from build123d import *

# Parameters (mm, degrees)
IZIM1_W                     = 30
IZIM1_H                     = 30
Y_KSEKLIK_EKSTR_ZYON1_DEPTH = 8
IZIM3_R                     = 1.75
KES_EKSTR_ZYON1_DEPTH       = 30
Y_KSEKLIK_EKSTR_ZYON3_DEPTH = 30
KES_EKSTR_ZYON2_DEPTH       = 30
IZIM5_R                     = 4.15
KES_EKSTR_ZYON3_DEPTH       = 30
IZIM6_W                     = 3
IZIM6_H                     = 1.5


with BuildPart() as part:
    # Çizim1 → Yükseklik-Ekstrüzyon1 (new body)
    with BuildSketch(Plane.XY):
        with Locations((15, 15)):
            Rectangle(IZIM1_W, IZIM1_H)
    extrude(amount=Y_KSEKLIK_EKSTR_ZYON1_DEPTH)

    # Çizim3 → Kes-Ekstrüzyon1 (cut)
    with BuildSketch(Plane.XY.offset(8)):
        with Locations((4, 26)):
            Circle(IZIM3_R)
        with Locations((4, 4)):
            Circle(IZIM3_R)
        with Locations((26, 26)):
            Circle(IZIM3_R)
        with Locations((26, 4)):
            Circle(IZIM3_R)
    extrude(amount=-KES_EKSTR_ZYON1_DEPTH, mode=Mode.SUBTRACT)

    # Çizim2 → Yükseklik-Ekstrüzyon3 (add)
    with BuildSketch(Plane.XY.offset(8)):
        with BuildLine():
            Line((6.161165235, 6.161165235), (9.590633124, 9.590633124))
            ThreePointArc((9.590633124, 9.590633124), (9.590633124, 20.409366876), (20.409366876, 20.409366876))
            Line((20.409366876, 20.409366876), (23.838834765, 23.838834765))
            ThreePointArc((23.838834765, 23.838834765), (6.161165235, 23.838834765), (6.161165235, 6.161165235))
        make_face()
    extrude(amount=Y_KSEKLIK_EKSTR_ZYON3_DEPTH)

    # Çizim4 → Kes-Ekstrüzyon2 (cut)
    with BuildSketch(Plane.XY.offset(8)):
        with BuildLine():
            Line((0, 15), (0, 30))
            Line((0, 30), (15, 30))
            ThreePointArc((15, 30), (6.161165235, 23.838834765), (0, 15))
        make_face()
    extrude(amount=-KES_EKSTR_ZYON2_DEPTH, mode=Mode.SUBTRACT)

    # Çizim5 → Kes-Ekstrüzyon3 (cut)
    with BuildSketch(Plane.XY.offset(8)):
        with Locations((15, 15)):
            Circle(IZIM5_R)
    extrude(amount=-KES_EKSTR_ZYON3_DEPTH, mode=Mode.SUBTRACT)

    # Çizim6 → Kes-Döndür1 (revolve, cut)
    with BuildSketch(Plane(origin=(0, 0, 0), x_dir=(0, 0, -1), z_dir=(0.7071067811865472, -0.7071067811865478, 0))):
        with Locations((-34.5, 32.963203436)):
            Rectangle(IZIM6_W, IZIM6_H)
        with Locations((-18, 32.963203436)):
            Rectangle(IZIM6_W, IZIM6_H)
    revolve(axis=Axis((15, 15, 42.321242124), (0, 0, -1)), mode=Mode.SUBTRACT)


solid = part.part
Geometry: final body of the model. Coordinates: model frame, mm. A direction names the side the tool comes from. Give positions to 0.01 mm unless a question says otherwise; leave off trailing zeros. Write each loop counter-clockwise with the first axis right and the second up, starting at its lowest first coordinate (ties: lowest second). Pieces come first, ordered by that corner, then holes. Notation, with made-up numbers: (72, 85.25) -> (124, 85.25) arc R29 cw to (124, 124.25) -> close; hole circle Ø3 at (22, 70). An arc over 180 degrees is marked (long way). Answer in a Markdown table with one row per item.
(1) Ray query, line 1 along Y through (x, z) = (26, 4); line 2 along Z through (x, y) = (19.5, 3.5); line 3 along X through (y, z) = (15, 17). Return the intervals inside material, ascending. Write a range as [from, to].
Answers below:
| item | result |
|---|---|
| line 1 | [0, 2.25], [5.75, 24.25], [27.75, 30] |
| line 2 | [0, 8] |
| line 3 | [4, 7.35] |
(2) Section query D-D on x = 21. Return loops of the section in (y, z).
Answers below:
| item | result |
|---|---|
| outline | (0, 0) -> (30, 0) -> (30, 8) -> (25.97, 8) -> (25.97, 16.5) -> (24.22, 16.5) -> (24.22, 19.5) -> (25.97, 19.5) -> (25.97, 33) -> (24.22, 33) -> (24.22, 36) -> (25.97, 36) -> (25.97, 38) -> (21, 38) -> (21, 8) -> (0, 8) -> close |
(3) Set-up query: faces 1 (the cylindrical face through (14.1, 10.95, 4.06)), 2 (the cylindrical face through (6.358, 24.031, 12.19)), 3 (the flat face through (0, 7, 4)), 4 (the cylindrical face through (7.053, 22.605, 17.979)), 5 (the flat face through (22, 22, 23)). Return all of +Z, -Z, +X, -X, +Y, -Y with unobstructed straight access to the full face (end or side cutting, diameter ignored); none if empty.
Answers below:
| item | result |
|---|---|
| face 1 | +Z, -Z |
| face 2 | +Z |
| face 3 | +Z, -Z, -X, +Y, -Y |
| face 4 | none |
| face 5 | +Z, +X, -Y |
(4) Draft query along X for faces 6 (the flat face through (22, 30, 4)), 7 (the cylindrical face through (6.269, 23.946, 4.056)), 8 (the cylindrical face through (9.473, 20.289, 22.79)). Return one class per face: +X half, -X half, draft (parallel to the pull), parting line (faces both ways), or undercut.
Answers below:
| item | result |
|---|---|
| face 6 | draft |
| face 7 | -X half |
| face 8 | undercut |
(5) Section query A-A on y = 4. Return loops of the section in (x, z), then the cut area to 3 significant figures.
Answers below:
| item | result |
|---|---|
| outline | (0, 0) -> (2.25, 0) -> (2.25, 8) -> (0, 8) -> close; (5.75, 0) -> (24.25, 0) -> (24.25, 8) -> (5.75, 8) -> close; (27.75, 0) -> (30, 0) -> (30, 8) -> (27.75, 8) -> close |
| area | 184 mm^2 |
(6) Section query B-B on z = 7. Return loops of the section in (x, y), then the cut area to 3 significant figures.
Answers below:
| item | result |
|---|---|
| outline | (0, 0) -> (30, 0) -> (30, 30) -> (15, 30) arc R30.66 ccw to (0, 15) -> close; hole circle Ø3.5 at (4, 4); hole circle Ø8.3 at (15, 15); hole circle Ø3.5 at (26, 4); hole circle Ø3.5 at (26, 26) |
| area | 731 mm^2 |
(7) Pin query (flat end, axial travel): pin 1 (8 mm diameter, centred on x = 15, z = 9.5, fed in from +Y); pin 2 (1 mm diameter, centred on y = 25, z = 34, fed in from +X); pin 3 (12 mm diameter, centred on x = 20.5, y = 4.5, fed in from +Z). Return the tip coordinate at first contact, or that it passes through.
Answers below:
| item | result |
|---|---|
| pin 1 | y = 30 |
| pin 2 | x = 20.55 |
| pin 3 | z = 8 |
